Work out the finished part from the listing and answer in its coordinate system (mm). Face numbers are marked on the shaded views. A direction names the side the tool comes from. Give positions to 0.01 mm unless a question says otherwise; leave off trailing zeros. Order: outer loops, then holes, each group sorted by start corner. A loop starts at its lowest first (then second) coordinate and runs counter-clockwise, first axis right, second up. Notation, with made-up numbers: (36.5, 79) -> (50.5, 79) arc R29 cw to (50.5, 108) -> close; hole circle Ø4 at (66, 29). An arc over 180 degrees is marked (long way). Answer as CSV lines item,"result". Start each with the question number.
1. Flat-ended cylindrical pins translate along their axes: pin 1 (0.7 mm diameter, centred on y = 16, z = 0.5, fed in from +X); pin 2 (1.5 mm diameter, centred on y = 15.5, z = 35, fed in from +X); pin 3 (1 mm diameter, centred on x = 154, z = 13, fed in from -Y); pin 4 (12 mm diameter, centred on y = -18.5, z = 16.5, fed in from +X). Find the tip coordinate at first contact, or state that the pin passes through.
2. For the marked faces 1, 2, 3 and 4, determine the directions among +Z, -Z, +X, -X, +Y, -Y from which every point of the face is accessible in a straight line to the end or side of a thin tool.
3. A cutting plane is placed at A-A (x = 0). Give the vertices of the cut face in (y, z).
4. For a pull along Y with two mould halves and no side action, classify the marked faces 5, 6, 7 and 8 as released by +Y, released by -Y, zero draft, split by the parting line, or undercut.
5. A cutting plane is placed at B-B (z = 18). Give the vertices of the cut face in (x, y).
6. A cutting plane is placed at D-D (x = 68). Give the vertices of the cut face in (y, z), then the cut area to 3 significant figures.
7. Find the intervals of material crossed by L1, parallel to Y at x = 0, z = 23; L2, parallel to Y at x = 40.5, z = 13; L3, parallel to X at y = 4.5, z = 32, in increasing order.
8. A cutting plane is placed at C-C (y = 0). Give the vertices of the cut face in (x, z).
from build123d import *

# Parameters (mm, degrees)
SKETCH_R        = 15
PAD_DEPTH       = 36
SKETCH001_R     = 15
PAD001_DEPTH    = 50
POCKET002_DEPTH = 45
FILLET_R        = 4
FILLET001_R     = 4


with BuildPart() as part:
    # Sketch → Pad (new body)
    with BuildSketch(Plane.XY):
        with BuildLine():
            ThreePointArc((20.021829, 22.341136), (-29.999994, 0.019609), (19.992607, -22.36729))
            ThreePointArc((35.300511, -16.52309), (27.107731, -18.033819), (19.992607, -22.36729))
            Line((35.300511, -16.52309), (125.352108, -16.52309))
            Line((125.352108, -16.52309), (125.352108, 16.47691))
            Line((125.352108, 16.47691), (35.352108, 16.47691))
            ThreePointArc((20.021829, 22.341136), (27.145303, 17.992999), (35.352108, 16.47691))
        make_face()
        Circle(SKETCH_R, mode=Mode.SUBTRACT)
    extrude(amount=PAD_DEPTH)

    # Sketch001 (on Face2 of Pad) → Pad001 (join)
    with BuildSketch(Plane.YZ.offset(125.352108)):
        with Locations((-0.02309, 18)):
            Circle(SKETCH001_R)
    extrude(amount=PAD001_DEPTH)

    # Sketch008 (on Face3 of Pad001) → Pocket002 (cut)
    with BuildSketch(Plane.YZ.offset(125.352108)):
        Polygon((-16.52309, 36), (-16.52309, 28.928932), (-9.452022, 36), align=None)
        Polygon((-16.52309, 7.071068), (-16.52309, 0), (-9.452022, 0), align=None)
        Polygon((16.52309, 28.975264), (9.452022, 36), (16.47691, 36), align=None)
        Polygon((9.405842, 0), (16.47691, 7.071068), (16.47691, 0), align=None)
    extrude(amount=-POCKET002_DEPTH, mode=Mode.SUBTRACT)

    # Fillet
    fillet_edges = [part.edges().sort_by_distance(p)[0] for p in [
        (80.352108, 12.964466, 32.51057),
        (80.352108, 12.941376, 3.535534),
    ]]
    fillet(fillet_edges, radius=FILLET_R)

    # Fillet001
    fillet001_edges = [part.edges().sort_by_distance(p)[0] for p in [
        (80.352108, -12.987556, 3.535534),
        (80.352108, -12.987556, 32.464466),
    ]]
    fillet(fillet001_edges, radius=FILLET001_R)


solid = part.part
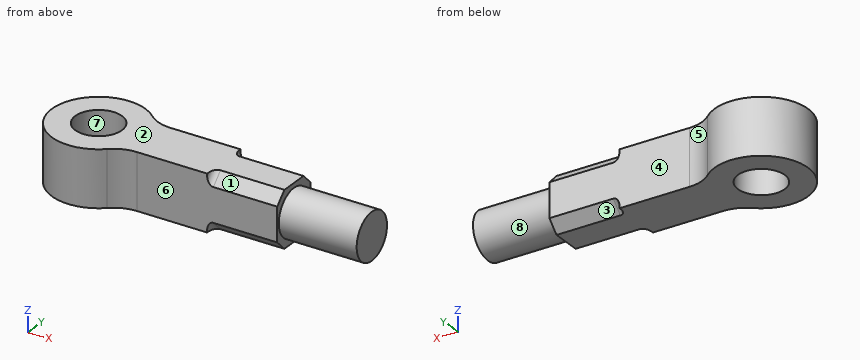
Answer sheet:
1,pin 1,"stops at x = 80.35"
1,pin 2,"stops at x = 80.54"
1,pin 3,"stops at y = -14.33"
1,pin 4,"stops at x = 175.35"
2,face 1,"+Z, +X, -Y"
2,face 2,"+Z, +X, -X, +Y, -Y"
2,face 3,"-Z, +X, +Y"
2,face 4,"+Z, -Z, +X, +Y"
3,outline,"(-30, 0) -> (-15, 0) -> (-15, 36) -> (-30, 36) -> close; (15, 0) -> (30, 0) -> (30, 36) -> (15, 36) -> close"
4,face 5,"released by +Y"
4,face 6,"released by -Y"
4,face 7,"undercut"
4,face 8,"split by the parting line"
5,outline,"(19.99, -22.37) arc R22.97 cw to (35.3, -16.52) -> (125.35, -16.52) -> (125.35, -15.02) -> (175.35, -15.02) -> (175.35, 14.98) -> (125.35, 14.98) -> (125.35, 16.48) -> (35.35, 16.48) arc R22.97 cw to (20.02, 22.34) arc R30 ccw (long way) to start; hole circle Ø30 at (0, 0)"
6,outline,"(-16.52, 0) -> (16.48, 0) -> (16.48, 36) -> (-16.52, 36) -> close"
6,area,"1,190 mm^2"
7,L1,"y = -30 to -15, 15 to 30"
7,L2,"y = -16.52 to 16.48"
7,L3,"x = -29.66 to -14.31, 14.31 to 175.35"
8,outline,"(-30, 0) -> (-15, 0) -> (-15, 36) -> (-30, 36) -> close; (15, 0) -> (125.35, 0) -> (125.35, 3) -> (175.35, 3) -> (175.35, 33) -> (125.35, 33) -> (125.35, 36) -> (15, 36) -> close"
